Can you work these out from the model? Positions are in its coordinate system, mm. A direction names the side the tool comes from. Give positions to 0.01 mm unless a question says otherwise; leave off trailing zeros. Loops run counter-clockwise (first coordinate to the right, second up) from the corner with the lowest first, then second, coordinate; pieces in that order, holes last. Notation, with made-up numbers: M -28,54 L 13,54 A16 ccw 13,60 Z; hole C 81.25,34.5 d1. An arc over 180 degrees is marked long. Put each result on its own line as item: value. Start each with the question number.
1) Imagine slicing it at A-A (z = 45.5). Write out the boundary of the cut face in (x, y).
2) For faces 5 (the flat face through (-80.5, 83.5, 84.71)), 6 (the flat face through (-93, 42.462, 64)), 7 (the flat face through (-93, 15.672, 63)), which set-ups out of +Z, -Z, +X, -X, +Y, -Y let a thin tool reach every point of the face, with its end or its side?
3) Please list where these lines run through material, in increasing order: line 1 along X through (y, z) = (25, 87); line 2 along Z through (x, y) = (-84, 22); line 3 along Z through (x, y) = (-93.5, 64.5). Write a range as from..to.
4) Imagine slicing it at C-C (y = 53.5). State how many separate pieces and enclosed holes the cut face has, then the cut area to 3 significant figures.
5) Imagine slicing it at D-D (z = 90). Write out the boundary of the cut face in (x, y), then the cut area to 3 significant figures.
6) For P1, Ø6, axis at x = -94, z = 14.5, coming from the -Y side; P2, Ø16, axis at x = -98, z = 68, coming from the -Y side; P3, Ø6, axis at x = -94.5, y = 66.5, coming from the +Z side; P4, Ø16, axis at x = -93.5, y = 23, coming from the +Z side, each with a flat end and sliding along its axis, tell me the tip position at first contact or that it passes through.
7) Imagine slicing it at B-B (x = -89). Write out the boundary of the cut face in (y, z), then the cut area to 3 significant figures.
8) If we mould it in two halves opening along X, with no side actions, what happens to faces 1 (the flat face through (-108.035, 52, 5)), 2 (the flat face through (-78.035, 51, 42)), 3 (the cylindrical face through (-105.56, 50.16, 94.88)), 4 (the flat face through (-103.025, 51, 48))? For each: +X half, -X half, draft (parallel to the pull), parting line (faces both ways), or undercut.
Solid Edge part; units mm, degrees
sketch "Sketch1" plane through (0, 0, 0) normal (0, 0, 1) x (1, 0, 0)
  line L0 (-108.0347, 1.2482) -> (-78.0347, 1.2482)
  line L1 (-78.0347, 1.2482) -> (-78.0347, 101.2482)
  line L2 (-78.0347, 101.2482) -> (-108.0347, 101.2482)
  line L3 (-108.0347, 101.2482) -> (-108.0347, 1.2482)
  dimension "D1" = 108.0347
  dimension "D2" = 78.0347
extrude "Protrusion1" add sketch "Sketch1" along normal blind 10
sketch "Sketch2" plane through (-78.0347, 51.2482, 5) normal (1, 0, 0) x (0, 1, 0)
  circle A0 centre (0, 85) radius 5
  line L0 (-50, 5) -> (-50, 55)
  line L1 (-50, 55) -> (-15, 103.734)
  line L2 (-15, 103.734) -> (15, 103.734)
  line L3 (15, 103.734) -> (50, 55)
  line L4 (50, 55) -> (50, 5)
  line L5 (50, 5) -> (-50, 5)
  dimension "D1" = 50
  dimension "D2" = 50
  dimension "D3" = 50
  dimension "D4" = 15
  dimension "D5" = 15
  dimension "D6" = 50
extrude "ExtrudedProtrusion_2" add sketch "Sketch2" against normal blind 5
mirror "Mirror1" about plane through (-93.03, 0, 0) normal (1, 0, 0) of "ExtrudedProtrusion_2"
sketch "Sketch3" plane through (-103.0253, 51.2482, 59.367) normal (1, 0, 0) x (0, 1, 0)
  line L0 (-35.5759, 20.7171) -> (-8.7862, 20.7171)
  line L1 (-8.7862, 20.7171) -> (-8.7862, -12.4376)
  line L2 (-8.7862, -12.4376) -> (-35.5759, -12.4376)
  line L3 (-35.5759, -12.4376) -> (-35.5759, 20.7171)
extrude "Protrusion3" add sketch "Sketch3" along normal up to vertex (19.9907 mm away)
Recorded:
1. outline: M -108.03,1.25 L -103.03,1.25 L -103.03,101.25 L -108.03,101.25 Z; M -83.03,1.25 L -78.03,1.25 L -78.03,101.25 L -83.03,101.25 Z
2. face 5: +Z, +X, -X, +Y
2. face 6: +Z, +Y
2. face 7: +Z, -Y
3. line 1: -108.03..-103.03, -83.03..-78.03
3. line 2: 0..10, 46.93..80.08
3. line 3: 0..10
4. separate pieces: 3
4. enclosed holes: 0
4. area: 1,200 mm²
5. outline: M -108.03,22.79 L -103.03,22.79 L -103.03,46.25 L -108.03,46.25 Z; M -108.03,56.25 L -103.03,56.25 L -103.03,79.7 L -108.03,79.7 Z; M -83.03,22.79 L -78.03,22.79 L -78.03,46.25 L -83.03,46.25 Z; M -83.03,56.25 L -78.03,56.25 L -78.03,79.7 L -83.03,79.7 Z
5. area: 469 mm²
6. P1: through
6. P2: y = 2.52
6. P3: z = 10
6. P4: z = 80.08
7. outline: M 1.25,0 L 101.25,0 L 101.25,10 L 1.25,10 Z; M 15.67,46.93 L 42.46,46.93 L 42.46,80.08 L 15.67,80.08 Z
7. area: 1,890 mm²
8. face 1: -X half
8. face 2: +X half
8. face 3: draft
8. face 4: undercut
